```python
from build123d import *

# Parameters (mm, degrees)
SKETCH1_W            = 96.4
SKETCH1_H            = 63
BOSS_EXTRUDE1_DEPTH  = 2.5
SKETCH1_5_W          = 93
SKETCH1_5_H          = 59.6
SKETCH1_5_W_2        = 86.9
SKETCH1_5_H_2        = 57
BOSS_EXTRUDE2_DEPTH  = 1.4
CHAMFER1_SIZE        = 1.5
SKETCH3_W            = 1.7
SKETCH3_H            = 13.2
BOSS_EXTRUDE4_DEPTH  = 1.7
SKETCH4_W            = 10
SKETCH4_H            = 1.7
SKETCH4_W_2          = 19.2
SKETCH4_W_3          = 13
BOSS_EXTRUDE5_DEPTH  = 1.6
SKETCH4_3_W          = 10
SKETCH4_3_H          = 1.7
SKETCH4_3_H_2        = 1.3
SKETCH4_3_W_2        = 19.2
SKETCH4_3_W_3        = 13
BOSS_EXTRUDE6_DEPTH  = 2
SKETCH3_5_W          = 3
SKETCH3_5_H          = 13.2
BOSS_EXTRUDE7_DEPTH  = 1
SKETCH5_W            = 1.7
SKETCH5_H            = 54.6
BOSS_EXTRUDE8_DEPTH  = 1.6
SKETCH5_3_W          = 1.3
SKETCH5_3_H          = 54.6
SKETCH5_3_W_2        = 1.7
BOSS_EXTRUDE9_DEPTH  = 2
SKETCH7_W            = 54.1
SKETCH7_H            = 8.9
CUT_EXTRUDE2_DEPTH   = 12
CHAMFER2_SIZE        = 1
SKETCH11_W           = 10
SKETCH11_H           = 2
SKETCH11_W_2         = 19.2
SKETCH11_W_3         = 13
BOSS_EXTRUDE10_DEPTH = 2
SKETCH13_W           = 10
SKETCH13_H           = 2
SKETCH13_W_2         = 19.2
SKETCH13_W_3         = 13
BOSS_EXTRUDE12_DEPTH = 0.9
SKETCH14_W           = 54.1
SKETCH14_H           = 3
BOSS_EXTRUDE13_DEPTH = 2.9
SKETCH15_W           = 2
SKETCH15_H           = 54.6
BOSS_EXTRUDE14_DEPTH = 4.5
SKETCH16_W           = 3.5
SKETCH16_H           = 54.6
BOSS_EXTRUDE15_DEPTH = 0.8
CUT_EXTRUDE3_DEPTH   = 10


with BuildPart() as part:
    # Sketch1 → Boss-Extrude1 (new body)
    with BuildSketch(Plane.XY):
        with Locations((10.058192988, -1.431154761)):
            Rectangle(SKETCH1_W, SKETCH1_H)
    extrude(amount=BOSS_EXTRUDE1_DEPTH)

    # Sketch1_5 → Boss-Extrude2 (add)
    # profile 1 of 2: a face of its own
    with BuildSketch(Plane.XY):
        with Locations((10.058192988, -1.431154761)):
            Rectangle(SKETCH1_5_W, SKETCH1_5_H)
        with Locations((11.808192988, -1.431154761)):
            Rectangle(SKETCH1_5_W_2, SKETCH1_5_H_2, mode=Mode.SUBTRACT)
    # profile 2 of 2: a face of its own
    with BuildSketch(Plane.XY):
        with Locations((11.808192988, -1.431154761)):
            Rectangle(SKETCH1_5_W_2, SKETCH1_5_H_2)
    extrude(amount=-BOSS_EXTRUDE2_DEPTH)

    # Chamfer1
    chamfer1_edges = [part.edges().sort_by_distance(p)[0] for p in [
        (-38.141807012, 30.068845239, 1.25),
        (58.258192988, 30.068845239, 1.25),
        (58.258192988, -32.931154761, 1.25),
        (-38.141807012, -32.931154761, 1.25),
    ]]
    chamfer(chamfer1_edges, length=CHAMFER1_SIZE)

    # Sketch3 → Boss-Extrude4 (add)
    with BuildSketch(Plane(origin=(0, 0, -1.4), x_dir=(-1, 0, 0), z_dir=(0, 0, -1))):
        with Locations((37.291807012, -1.631154761)):
            Rectangle(SKETCH3_W, SKETCH3_H)
    extrude(amount=-BOSS_EXTRUDE4_DEPTH)

    # Sketch4 → Boss-Extrude5 (add)
    with BuildSketch(Plane(origin=(0, 0, -1.4), x_dir=(-1, 0, 0), z_dir=(0, 0, -1))):
        with Locations((-22.068192988, 29.218845239)):
            Rectangle(SKETCH4_W, SKETCH4_H)
        with Locations((-0.358192988, 29.218845239)):
            Rectangle(SKETCH4_W_2, SKETCH4_H)
        with Locations((20.741807012, 29.218845239)):
            Rectangle(SKETCH4_W_3, SKETCH4_H)
    extrude(amount=-BOSS_EXTRUDE5_DEPTH)

    # Sketch4_3 → Boss-Extrude6 (add)
    with BuildSketch(Plane(origin=(0, 0, -1.4), x_dir=(-1, 0, 0), z_dir=(0, 0, -1))):
        with Locations((-22.068192988, 29.218845239)):
            Rectangle(SKETCH4_3_W, SKETCH4_3_H)
        with Locations((-22.068192988, 27.718845239)):
            Rectangle(SKETCH4_3_W, SKETCH4_3_H_2)
        with Locations((-0.358192988, 27.718845239)):
            Rectangle(SKETCH4_3_W_2, SKETCH4_3_H_2)
        with Locations((-0.358192988, 29.218845239)):
            Rectangle(SKETCH4_3_W_2, SKETCH4_3_H)
        with Locations((20.741807012, 27.718845239)):
            Rectangle(SKETCH4_3_W_3, SKETCH4_3_H_2)
        with Locations((20.741807012, 29.218845239)):
            Rectangle(SKETCH4_3_W_3, SKETCH4_3_H)
    extrude(amount=BOSS_EXTRUDE6_DEPTH)

    # Sketch3_5 → Boss-Extrude7 (add)
    with BuildSketch(Plane(origin=(0, 0, -1.4), x_dir=(-1, 0, 0), z_dir=(0, 0, -1))):
        with Locations((36.641807012, -1.631154761)):
            Rectangle(SKETCH3_5_W, SKETCH3_5_H)
    extrude(amount=BOSS_EXTRUDE7_DEPTH)

    # Sketch5 → Boss-Extrude8 (add)
    with BuildSketch(Plane(origin=(0, 0, -1.4), x_dir=(-1, 0, 0), z_dir=(0, 0, -1))):
        with Locations((-57.408192988, -2.231154761)):
            Rectangle(SKETCH5_W, SKETCH5_H)
    extrude(amount=-BOSS_EXTRUDE8_DEPTH)

    # Sketch5_3 → Boss-Extrude9 (add)
    with BuildSketch(Plane(origin=(0, 0, -1.4), x_dir=(-1, 0, 0), z_dir=(0, 0, -1))):
        with Locations((-55.908192988, -2.231154761)):
            Rectangle(SKETCH5_3_W, SKETCH5_3_H)
        with Locations((-57.408192988, -2.231154761)):
            Rectangle(SKETCH5_3_W_2, SKETCH5_3_H)
    extrude(amount=BOSS_EXTRUDE9_DEPTH)

    # Sketch7 → Cut-Extrude2 (cut)
    with BuildSketch(Plane.XY.offset(2.5)):
        with Locations((1.008192988, -25.481154761)):
            Rectangle(SKETCH7_W, SKETCH7_H)
    extrude(amount=-CUT_EXTRUDE2_DEPTH, mode=Mode.SUBTRACT)

    # Chamfer2
    chamfer2_edges = [part.edges().sort_by_distance(p)[0] for p in [
        (28.058192988, -29.931154761, 0.55),
        (-26.041807012, -29.931154761, 0.55),
        (-26.041807012, -21.031154761, 0.55),
        (28.058192988, -21.031154761, 0.55),
    ]]
    chamfer(chamfer2_edges, length=CHAMFER2_SIZE)

    # Sketch11 → Boss-Extrude10 (add)
    with BuildSketch(Plane.XZ.offset(-27.068845239)):
        with Locations((22.068192988, -2.4)):
            Rectangle(SKETCH11_W, SKETCH11_H)
        with Locations((0.358192988, -2.4)):
            Rectangle(SKETCH11_W_2, SKETCH11_H)
        with Locations((-20.741807012, -2.4)):
            Rectangle(SKETCH11_W_3, SKETCH11_H)
    extrude(amount=BOSS_EXTRUDE10_DEPTH)

    # Sketch13 → Boss-Extrude12 (add)
    with BuildSketch(Plane(origin=(0, 0, -3.4), x_dir=(-1, 0, 0), z_dir=(0, 0, -1))):
        with Locations((-22.068192988, 26.068845239)):
            Rectangle(SKETCH13_W, SKETCH13_H)
        with Locations((-0.358192988, 26.068845239)):
            Rectangle(SKETCH13_W_2, SKETCH13_H)
        with Locations((20.741807012, 26.068845239)):
            Rectangle(SKETCH13_W_3, SKETCH13_H)
    extrude(amount=BOSS_EXTRUDE12_DEPTH)

    # Sketch14 → Boss-Extrude13 (add)
    with BuildSketch(Plane(origin=(0, 0, -1.4), x_dir=(-1, 0, 0), z_dir=(0, 0, -1))):
        with Locations((-1.008192988, -19.531154761)):
            Rectangle(SKETCH14_W, SKETCH14_H)
    extrude(amount=BOSS_EXTRUDE13_DEPTH)

    # Sketch15 → Boss-Extrude14 (add)
    with BuildSketch(Plane.ZY.offset(-55.258192988)):
        with Locations((-2.4, -2.231154761)):
            Rectangle(SKETCH15_W, SKETCH15_H)
    extrude(amount=BOSS_EXTRUDE14_DEPTH)

    # Sketch16 → Boss-Extrude15 (add)
    with BuildSketch(Plane(origin=(0, 0, -3.4), x_dir=(-1, 0, 0), z_dir=(0, 0, -1))):
        with Locations((-52.508192988, -2.231154761)):
            Rectangle(SKETCH16_W, SKETCH16_H)
    extrude(amount=BOSS_EXTRUDE15_DEPTH)

    # Sketch17 → Cut-Extrude3 (cut)
    with BuildSketch(Plane.XY.offset(2.5)):
        with BuildLine():
            Line((3.271081669, 1.417718204), (3.271081669, -13.776270945))
            ThreePointArc((3.271081669, -13.776270945), (4.722208704, -15.227397979), (6.173335738, -13.776270945))
            Line((6.173335738, -13.776270945), (6.173335738, 1.417718204))
            ThreePointArc((6.173335738, 1.417718204), (4.722208704, 2.868845239), (3.271081669, 1.417718204))
        make_face()
        with BuildLine():
            Line((15.271081669, 1.417718204), (15.271081669, -13.776270945))
            ThreePointArc((15.271081669, -13.776270945), (16.722208704, -15.227397979), (18.173335738, -13.776270945))
            Line((18.173335738, -13.776270945), (18.173335738, 1.417718204))
            ThreePointArc((18.173335738, 1.417718204), (16.722208704, 2.868845239), (15.271081669, 1.417718204))
        make_face()
        with BuildLine():
            Line((9.271081669, 1.417718204), (9.271081669, -13.776270945))
            ThreePointArc((9.271081669, -13.776270945), (10.722208704, -15.227397979), (12.173335738, -13.776270945))
            Line((12.173335738, -13.776270945), (12.173335738, 1.417718204))
            ThreePointArc((12.173335738, 1.417718204), (10.722208704, 2.868845239), (9.271081669, 1.417718204))
        make_face()
    extrude(amount=-CUT_EXTRUDE3_DEPTH, mode=Mode.SUBTRACT)


solid = part.part
```
Input: part model. Units: mm. Frame: model coordinates. A direction names the side the tool comes from. Give positions to 0.01 mm unless a question says otherwise; leave off trailing zeros. Loops run counter-clockwise (first coordinate to the right, second up) from the corner with the lowest first, then second, coordinate; pieces in that order, holes last. Notation, with made-up numbers: (-23, 1) -> (32, 1) arc R8 cw to (32, 16) -> close; hole circle Ø11 at (-33.5, -25.5). An arc over 180 degrees is marked (long way). Use a Markdown table: item, result.
Q1. Section query A-A, the plane x = -6. Return the cut outline in (y, z), plus the area to 3 significant figures.
Entries:
| item | result |
|---|---|
| outline | (-32.93, 0) -> (-31.23, 0) -> (-31.23, -1.4) -> (-29.93, -1.4) -> (-29.93, 2.5) -> (-32.93, 2.5) -> close; (-21.03, -4.3) -> (-18.03, -4.3) -> (-18.03, -1.4) -> (25.07, -1.4) -> (25.07, -4.3) -> (27.07, -4.3) -> (27.07, -3.4) -> (30.07, -3.4) -> (30.07, 2.5) -> (-21.03, 2.5) -> close |
| area | 229 mm² |
Q2. Ray query, probe 1 along X at (y, z) = (-6, 0); probe 2 along X at (y, z) = (-10, -1); probe 3 along Y at (x, z) = (-1, -1.25). Return the intervals inside material, ascending. Write a range as from..to.
Entries:
| item | result |
|---|---|
| probe 1 | x = -38.14..3.27, 6.17..9.27, 12.17..15.27, 18.17..58.26 |
| probe 2 | x = -36.44..3.27, 6.17..9.27, 12.17..15.27, 18.17..58.26 |
| probe 3 | y = -31.23..-29.93, -21.03..30.07 |
Q3. Section query D-D, the plane y = 21.5. Return the cut outline in (x, z).
Entries:
| item | result |
|---|---|
| outline | (-38.14, 0) -> (-36.44, 0) -> (-36.44, -1.4) -> (50.76, -1.4) -> (50.76, -4.2) -> (54.26, -4.2) -> (54.26, -3.4) -> (58.26, -3.4) -> (58.26, 2.5) -> (-38.14, 2.5) -> close |
Q4. Section query C-C, the plane y = -24. Return the cut outline in (x, z).
Entries:
| item | result |
|---|---|
| outline | (-38.14, 0) -> (-36.44, 0) -> (-36.44, -1.4) -> (-26.04, -1.4) -> (-26.04, 2.5) -> (-38.14, 2.5) -> close; (28.06, -1.4) -> (50.76, -1.4) -> (50.76, -4.2) -> (54.26, -4.2) -> (54.26, -3.4) -> (58.26, -3.4) -> (58.26, 2.5) -> (28.06, 2.5) -> close |
Q5. First-contact query: P1, Ø0.9, axis at y = -16, z = -4, coming from the +X side; P2, Ø3, axis at x = 2, z = -3, coming from the -Y side; P3, Ø3, axis at x = 2, z = -2, coming from the -Y side; P4, Ø5, axis at x = -5.5, y = -26.5, coming from the +Z side. Flat tips, straight axial feed; report the tip coordinate or a pass-through.
Entries:
| item | result |
|---|---|
| P1 | stops at x = 54.26 |
| P2 | stops at y = -21.03 |
| P3 | stops at y = -31.23 |
| P4 | passes through |
Q6. Access query for faces 1 (the flat face through (-9.242, 28, -2)), 2 (the flat face through (0, 25.069, -3)), 3 (the cylindrical face through (10.69, -15.227, 0.577)). Directions: +Z, -Z, +X, -X, +Y, -Y. A direction counts if a zero-diameter tool reaches every point of the face in a straight line with its end or side. Return the directions, or none.
Entries:
| item | result |
|---|---|
| face 1 | -Z, +Y |
| face 2 | -Z, -X |
| face 3 | +Z, -Z |
Q7. Section query B-B, the plane y = -12. Return the cut outline in (x, z), plus the area to 3 significant figures.
Entries:
| item | result |
|---|---|
| outline | (-38.14, 0) -> (-36.44, 0) -> (-36.44, -1.4) -> (3.27, -1.4) -> (3.27, 2.5) -> (-38.14, 2.5) -> close; (6.17, -1.4) -> (9.27, -1.4) -> (9.27, 2.5) -> (6.17, 2.5) -> close; (12.17, -1.4) -> (15.27, -1.4) -> (15.27, 2.5) -> (12.17, 2.5) -> close; (18.17, -1.4) -> (50.76, -1.4) -> (50.76, -4.2) -> (54.26, -4.2) -> (54.26, -3.4) -> (58.26, -3.4) -> (58.26, 2.5) -> (18.17, 2.5) -> close |
| area | 357 mm² |
Q8. Pull-direction query (Y, two-part tool) for faces 4 (the flat face through (28.058, -20, -3)), 5 (the flat face through (1, -21.031, -1)); classes: pulls with the +Y half, pulls with the -Y half, needs draft (parallel to the pull), parting line crosses it, or undercut.
Entries:
| item | result |
|---|---|
| face 4 | needs draft |
| face 5 | undercut |
